```python
from build123d import *

# Parameters (mm, degrees)
SKETCH1_R           = 11.43
BOSS_EXTRUDE1_DEPTH = 0.254
SKETCH2_R           = 3.683
SKETCH2_R_2         = 3.556
BOSS_EXTRUDE2_DEPTH = 62.992
SKETCH3_R           = 11.43
BOSS_EXTRUDE3_DEPTH = 0.254
SKETCH5_W           = 43.942
SKETCH5_H           = 2.032
CUT_EXTRUDE1_DEPTH  = 2.794
SKETCH6_W           = 34.798
SKETCH6_H           = 1.980001403
CUT_EXTRUDE3_DEPTH  = 2.794
SKETCH7_R           = 2.032
CUT_EXTRUDE4_DEPTH  = 64.5


with BuildPart() as part:
    # Sketch1 → Boss-Extrude1 (new body)
    with BuildSketch(Plane(origin=(0, 0, 0), x_dir=(0, 0, -1), z_dir=(1, 0, 0))):
        Circle(SKETCH1_R)
    extrude(amount=BOSS_EXTRUDE1_DEPTH)

    # Sketch2 → Boss-Extrude2 (add)
    with BuildSketch(Plane(origin=(0.254, 0, 0), x_dir=(0, 0, -1), z_dir=(1, 0, 0))):
        Circle(SKETCH2_R)
        Circle(SKETCH2_R_2, mode=Mode.SUBTRACT)
    extrude(amount=BOSS_EXTRUDE2_DEPTH)

    # Sketch3 → Boss-Extrude3 (add)
    with BuildSketch(Plane(origin=(63.246, 0, 0), x_dir=(0, 0, -1), z_dir=(1, 0, 0))):
        Circle(SKETCH3_R)
    extrude(amount=BOSS_EXTRUDE3_DEPTH)

    # Sketch5 → Cut-Extrude1 (cut)
    with BuildSketch(Plane.XY.offset(3.683)):
        with Locations((31.75, 0)):
            Rectangle(SKETCH5_W, SKETCH5_H)
    extrude(amount=-CUT_EXTRUDE1_DEPTH, mode=Mode.SUBTRACT)

    # Sketch6 → Cut-Extrude3 (cut)
    with BuildSketch(Plane.XY.offset(-3.683)):
        with Locations((31.75, 0.025999298)):
            Rectangle(SKETCH6_W, SKETCH6_H)
    extrude(amount=CUT_EXTRUDE3_DEPTH, mode=Mode.SUBTRACT)

    # Sketch7 → Cut-Extrude4 (cut, through all)
    with BuildSketch(Plane(origin=(63.5, 0, 0), x_dir=(0, 0, -1), z_dir=(1, 0, 0))):
        with BuildLine():
            Line((-2.667, -1.016), (-1.75976362, -1.016))
            ThreePointArc((-1.75976362, -1.016), (-2.032, 0), (-1.75976362, 1.016))
            Line((-1.75976362, 1.016), (-2.667, 1.016))
            ThreePointArc((-2.667, 1.016), (-3.026210245, 0.867210245), (-3.175, 0.508))
            Line((-3.175, 0.508), (-3.175, -0.508))
            ThreePointArc((-3.175, -0.508), (-3.026210245, -0.867210245), (-2.667, -1.016))
        make_face()
        with BuildLine():
            ThreePointArc((2.667, -1.016), (3.026210245, -0.867210245), (3.175, -0.508))
            Line((3.175, -0.508), (3.175, 0.508))
            ThreePointArc((3.175, 0.508), (3.026210245, 0.867210245), (2.667, 1.016))
            Line((2.667, 1.016), (1.75976362, 1.016))
            ThreePointArc((1.75976362, 1.016), (1.962761279, 0.5259203), (2.032, 0))
            ThreePointArc((2.032, 0), (1.962761279, -0.5259203), (1.75976362, -1.016))
            Line((1.75976362, -1.016), (2.667, -1.016))
        make_face()
        Circle(SKETCH7_R)
    extrude(amount=-CUT_EXTRUDE4_DEPTH, mode=Mode.SUBTRACT)


solid = part.part
```
Geometry check sheet. Reference: the model listing, model coordinates, mm. Round coordinates to 2 decimals unless told otherwise and drop trailing zeros. Loops run counter-clockwise (first coordinate to the right, second up) from the corner with the lowest first, then second, coordinate; pieces in that order, holes last. Notation, with made-up numbers: (85.5, -5.5) -> (121.5, -5.5) arc R17 ccw to (121.5, 9.5) -> close; hole circle Ø9 at (0, -37). An arc over 180 degrees is marked (long way). Use a Markdown table: item, result.
(1) Sectioned sample at B-B (x = 38). Enter the section's corners in (y, z), then the cut area to 3 significant figures.
Calculated:
| item | result |
|---|---|
| outline | (-1.02, 3.41) -> (-1.02, 3.54) arc R3.68 ccw to (-0.96, -3.55) -> (-0.96, -3.42) arc R3.56 cw to start; (1.02, -3.54) arc R3.68 ccw to (1.02, 3.54) -> (1.02, 3.41) arc R3.56 cw to (1.02, -3.41) -> close |
| area | 2.37 mm² |
(2) Sectioned sample at A-A (z = 0). Enter the section's corners in (x, y).
Calculated:
| item | result |
|---|---|
| outline | (0, -11.43) -> (0.25, -11.43) -> (0.25, -3.68) -> (63.25, -3.68) -> (63.25, -11.43) -> (63.5, -11.43) -> (63.5, -2.03) -> (63.25, -2.03) -> (63.25, -3.56) -> (0.25, -3.56) -> (0.25, -2.03) -> (0, -2.03) -> close; (0, 2.03) -> (0.25, 2.03) -> (0.25, 3.56) -> (63.25, 3.56) -> (63.25, 2.03) -> (63.5, 2.03) -> (63.5, 11.43) -> (63.25, 11.43) -> (63.25, 3.68) -> (0.25, 3.68) -> (0.25, 11.43) -> (0, 11.43) -> close |
(3) Sectioned sample at C-C (y = 8.25). Enter the section's corners in (x, z), then the cut area to 3 significant figures.
Calculated:
| item | result |
|---|---|
| outline | (0, -7.91) -> (0.25, -7.91) -> (0.25, 7.91) -> (0, 7.91) -> close; (63.25, -7.91) -> (63.5, -7.91) -> (63.5, 7.91) -> (63.25, 7.91) -> close |
| area | 8.04 mm² |
(4) Sectioned sample at D-D (x = 11). Enter the section's corners in (y, z).
Calculated:
| item | result |
|---|---|
| outline | (-1.02, 3.41) -> (-1.02, 3.54) arc R3.68 ccw (long way) to (1.02, 3.54) -> (1.02, 3.41) arc R3.56 cw (long way) to start |
(5) Mould release check, pull along X, two halves, no side actions. Record for faces 1 (the flat face through (0, -2.4, 0.2)), 2 (the flat face through (63.246, 3, 3)), 3 (the flat face through (63.5, -2.4, 0.2)): released by +X, released by -X, zero draft, split by the parting line, or undercut.
Calculated:
| item | result |
|---|---|
| face 1 | released by -X |
| face 2 | undercut |
| face 3 | released by +X |
(6) Go/stop test with flat-tipped pins: P1, Ø2, axis at x = 54.5, z = -6.5, coming from the -Y side; P2, Ø1, axis at x = 6.5, y = -3, coming from the -Z side; P3, Ø2, axis at x = 25, z = 2.5, coming from the +Y side; P4, Ø8, axis at x = 9.5, z = -2, coming from the -Y side. Record where each tip stops, or that it passes through.
Calculated:
| item | result |
|---|---|
| P1 | through |
| P2 | z = -2.7 |
| P3 | y = 3.36 |
| P4 | y = -3.68 |
(7) Scan lines: probe 1 along X at (y, z) = (-8.25, -0.5); probe 2 along Z at (x, y) = (8, 3.25); probe 3 along Z at (x, y) = (26.5, -2.25). Record each from-to range of solid material in increasing order.
Calculated:
| item | result |
|---|---|
| probe 1 | 0 to 0.25, 63.25 to 63.5 |
| probe 2 | -1.73 to -1.44, 1.44 to 1.73 |
| probe 3 | -2.92 to -2.75, 2.75 to 2.92 |
